from build123d import *

# Parameters (mm, degrees)
SKETCH_5_W      = 8.106936937
SKETCH_5_H      = 24.2
EXTRUDE_3_DEPTH = 2


with BuildPart() as part:
    # 스케치5 → 보스-돌출3 (new body)
    with BuildSketch(Plane(origin=(0, 0, 0), x_dir=(1, 0, 0), z_dir=(0, 1, 0))):
        with Locations((2.053468469, -10)):
            Rectangle(SKETCH_5_W, SKETCH_5_H)
        Polygon((-0.1, -13.871307421), (1.399695667, -10), (-0.1, -6.128692579), (-0.1, 0.1), (1.068502531, 0.1), (3.005439468, -4.9), (4.106936937, -4.9), (4.106936937, -15.1), (3.005439468, -15.1), (1.068502531, -20.1), (-0.1, -20.1), align=None, mode=Mode.SUBTRACT)
    extrude(amount=EXTRUDE_3_DEPTH)


solid = part.part
Read the model definition and answer for the solid it produces. Units are mm, in the model's axes. A direction names the side the tool comes from. Give positions to 0.01 mm unless a question says otherwise; leave off trailing zeros. Write each loop counter-clockwise with the first axis right and the second up, starting at its lowest first coordinate (ties: lowest second). Pieces come first, ordered by that corner, then holes. Notation, with made-up numbers: (-18.5, 9) - (38.5, 9) arc R24 ccw to (38.5, 33) - close; hole circle Ø3 at (-39.5, 46). An arc over 180 degrees is marked (long way). Answer in a Markdown table with one row per item. Add a question column.
Item 1: A tool of negligible diameter and unlimited length cuts with its end or side. For faces 4 (the face through (2.05, 0.99, 17.57)), 5 (the face through (1, 0, 10)), from which of +Z, -Z, +X, -X, +Y, -Y can it reach the whole face along a straight path? Write none if from no direction.
Item 2: Section A-A, the plane y = 0.8 is taken. Write down the section's boundary in (x, z).
Item 3: Find the intervals of material crossed by L1, parallel to X at y = 1, z = 0.75; L2, parallel to X at y = 0.4, z = 5.5; L3, parallel to Z at x = 3.25, y = 1.6, in increasing order.
Item 4: Determine the mould class of faces 1 (the face through (2, 1, -2.1)), 2 (the face through (6.107, 1, 10)), 3 (the face through (-0.1, 1, 17)) for opening direction X: pulls with the +X half, pulls with the -X half, needs draft (parallel to the pull), parting line crosses it, or undercut.
Item 5: Section C-C, the plane x = 2 is taken. Write down the section's boundary in (y, z).
Item 6: Section B-B, the plane z = 8 is taken. Write down the section's boundary in (x, y), and give its area (3 significant figures).
Item 7: A flat-ended cylindrical pin translates along its axis: P1, Ø2, axis at x = 2.5, z = 12, coming from the +Y side. Find the tip coordinate at first contact, or state that the pin passes through.
Recorded:
| question | item | result |
|---|---|---|
| 1 | face 4 | +Y, -Y |
| 1 | face 5 | +Z, -Z, +X, -X, -Y |
| 2 | outline | (-2, -2.1) - (6.11, -2.1) - (6.11, 22.1) - (-2, 22.1) - close; hole (-0.1, -0.1) - (1.07, -0.1) - (3.01, 4.9) - (4.11, 4.9) - (4.11, 15.1) - (3.01, 15.1) - (1.07, 20.1) - (-0.1, 20.1) - (-0.1, 13.87) - (1.4, 10) - (-0.1, 6.13) - close |
| 3 | L1 | x = -2 to -0.1, 1.4 to 6.11 |
| 3 | L2 | x = -2 to -0.1, 4.11 to 6.11 |
| 3 | L3 | z = -2.1 to 4.9, 15.1 to 22.1 |
| 4 | face 1 | needs draft |
| 4 | face 2 | pulls with the +X half |
| 4 | face 3 | undercut |
| 5 | outline | (0, -2.1) - (2, -2.1) - (2, 2.3) - (0, 2.3) - close; (0, 17.7) - (2, 17.7) - (2, 22.1) - (0, 22.1) - close |
| 6 | outline | (-2, 0) - (0.62, 0) - (0.62, 2) - (-2, 2) - close; (4.11, 0) - (6.11, 0) - (6.11, 2) - (4.11, 2) - close |
| 6 | area | 9.25 mm2 |
| 7 | P1 | passes through |
